Work out the finished part from the listing and answer in its coordinate system (mm). Give positions to 0.01 mm unless a question says otherwise; leave off trailing zeros. Loops run counter-clockwise (first coordinate to the right, second up) from the corner with the lowest first, then second, coordinate; pieces in that order, holes last. Notation, with made-up numbers: (1, 87) - (11, 87) arc R27 cw to (11, 108) - close; hole circle Ø3 at (46.5, -9). An arc over 180 degrees is marked (long way). One line per item, written item: value.
Autodesk Inventor part; units mm, degrees
ref_plane "YZ Plane" through (0, 0, 0) normal (1, 0, 0) x (0, 1, 0)
ref_plane "XZ Plane" through (0, 0, 0) normal (0, 1, 0) x (-1, 0, 0)
ref_plane "XY Plane" through (0, 0, 0) normal (0, 0, 1) x (1, 0, 0)
sketch "Sketch1" plane through (0, 0, 0) normal (0, 0, 1) x (1, 0, 0)
  line L0 (-5.04, 3.6) -> (5.04, 3.6)
  line L1 (5.04, 3.6) -> (5.04, -3.6)
  line L2 (-5.04, -3.6) -> (-5.04, 3.6)
  line L3 (-2.79, -3.4) -> (-2.79, -3.6)
  line L4 (-2.79, -3.6) -> (-2.29, -3.6)
  line L5 (-2.29, -3.6) -> (-2.29, -3.4)
  line L6 (-0.25, -3.4) -> (-0.25, -3.6)
  line L7 (-0.25, -3.6) -> (0.25, -3.6)
  line L8 (0.25, -3.6) -> (0.25, -3.4)
  line L9 (2.29, -3.4) -> (2.29, -3.6)
  line L10 (2.29, -3.6) -> (2.79, -3.6)
  line L11 (2.79, -3.6) -> (2.79, -3.4)
  line L12 (-2.79, -3.4) -> (-4.79, -3.4)
  line L13 (-0.25, -3.4) -> (-2.29, -3.4)
  line L14 (4.79, -3.4) -> (2.79, -3.4)
  line L15 (2.29, -3.4) -> (0.25, -3.4)
  line L16 (0, 1.3653) -> (0, -1.7187) construction
  line L17 (-4.79, -3.4) -> (-4.79, -3.6)
  line L18 (-4.79, -3.6) -> (-5.04, -3.6)
  line L19 (4.79, -3.4) -> (4.79, -3.6)
  line L20 (4.79, -3.6) -> (5.04, -3.6)
  point P0 (0, 0)
  point P1 (0, 3.6)
  point P2 (-5.04, 0)
  point P3 (0, -3.6)
  point P4 (-2.54, -3.6)
  point P5 (-2.54, -3.6)
  point P6 (5.04, 0)
  dimension "d0" = 0.5
  dimension "d1" = 0.2
  dimension "d3" = 10.08
  dimension "d4" = 2.54
  dimension "d20" = 7
  dimension "d21" = 0.25
extrude "Extrusion1" add sketch "Sketch1" along normal blind 2.54
sketch "Sketch3" plane through (-5.04, -3.4, 0) normal (0, -1, 0) x (1, 0, 0)
  line L0 (0.93, 2.87) -> (1.53, 2.87)
  line L1 (1.53, 2.87) -> (1.53, 1.87)
  line L2 (1.53, 1.87) -> (0.93, 1.87)
  line L3 (0.93, 1.87) -> (0.93, 2.87)
  line L4 (0.93, 0.67) -> (1.53, 0.67)
  line L5 (1.53, 0.67) -> (1.53, -0.33)
  line L6 (1.53, -0.33) -> (0.93, -0.33)
  line L7 (0.93, -0.33) -> (0.93, 0.67)
  line L8 (3.47, 2.87) -> (4.07, 2.87)
  line L9 (4.07, 2.87) -> (4.07, 1.87)
  line L10 (4.07, 1.87) -> (3.47, 1.87)
  line L11 (3.47, 1.87) -> (3.47, 2.87)
  line L12 (3.47, 0.67) -> (4.07, 0.67)
  line L13 (4.07, 0.67) -> (4.07, -0.33)
  line L14 (4.07, -0.33) -> (3.47, -0.33)
  line L15 (3.47, -0.33) -> (3.47, 0.67)
  line L16 (6.01, 2.87) -> (6.61, 2.87)
  line L17 (6.61, 2.87) -> (6.61, 1.87)
  line L18 (6.61, 1.87) -> (6.01, 1.87)
  line L19 (6.01, 1.87) -> (6.01, 2.87)
  line L20 (6.01, 0.67) -> (6.61, 0.67)
  line L21 (6.61, 0.67) -> (6.61, -0.33)
  line L22 (6.61, -0.33) -> (6.01, -0.33)
  line L23 (6.01, -0.33) -> (6.01, 0.67)
  line L24 (8.55, 2.87) -> (9.15, 2.87)
  line L25 (9.15, 2.87) -> (9.15, 1.87)
  line L26 (9.15, 1.87) -> (8.55, 1.87)
  line L27 (8.55, 1.87) -> (8.55, 2.87)
  line L28 (8.55, 0.67) -> (9.15, 0.67)
  line L29 (9.15, 0.67) -> (9.15, -0.33)
  line L30 (9.15, -0.33) -> (8.55, -0.33)
  line L31 (8.55, -0.33) -> (8.55, 0.67)
  line L32 (4.79, 0) -> (2.75, 0)
  line L33 (6.0777, 1.27) -> (8.8799, 1.27) construction
  line L34 (0, 0) -> (0, 2.54)
  line L35 (0, 0) -> (0, 2.54)
  point P0 (5.04, 0)
  point P1 (1.23, -0.33)
  point P2 (3.77, -0.33)
  point P3 (6.31, -0.33)
  point P4 (8.85, -0.33)
  point P5 (3.77, -0.33)
  point P6 (1.23, -0.33)
  point P7 (6.31, -0.33)
  point P8 (8.85, -0.33)
  point P9 (3.77, 0)
  point P10 (0, 1.27)
  dimension "d11" = 3.2
  dimension "d12" = 0.6
  dimension "d13" = 2.54
  dimension "d14" = 2.54
  dimension "d15" = 2.54
  dimension "d16" = 1
extrude "Extrusion3" add sketch "Sketch3" along normal blind 0.2
sketch "Sketch5" plane through (-5.04, 3.6, 0) normal (0, 1, 0) x (1, 0, 0)
  line L0 (0, 0) -> (10.08, 0)
  line L1 (0, 0) -> (0, -2.54)
  line L2 (10.08, -2.54) -> (0, -2.54)
  line L3 (10.08, 0) -> (10.08, -2.54)
  line L4 (0.73, -0.77) -> (1.73, -0.77)
  line L5 (1.73, -0.77) -> (1.73, -1.77)
  line L6 (1.73, -1.77) -> (0.73, -1.77)
  line L7 (0.73, -1.77) -> (0.73, -0.77)
  line L8 (1.53, 0.33) -> (0.93, 0.33)
  point P0 (5.04, 0)
  point P1 (0.73, -1.27)
  point P2 (0, -1.27)
  point P3 (1.23, -0.77)
  point P4 (1.23, 0.33)
  dimension "d23" = 1
extrude "Extrusion4" cut sketch "Sketch5" against normal blind 7 contours L4 L5 L6 L7
chamfer "Chamfer1" distance 0.5 angle 45 4 edges at (-3.81, 3.6, 0.77) (-3.31, 3.6, 1.27) (-4.31, 3.6, 1.27) (-3.81, 3.6, 1.77)
pattern_linear "Rectangular Pattern1" count 4 spacing 2.54 along (1, 0, 0) of "Extrusion4", "Chamfer1"
properties part number "fciconnect-91601-304"
1. Section A-A (y = -3) is taken. Write down the section's boundary in (x, z).
Output:
outline: (-5.04, 0) - (5.04, 0) - (5.04, 2.54) - (-5.04, 2.54) - close; hole (-4.31, 0.77) - (-3.31, 0.77) - (-3.31, 1.77) - (-4.31, 1.77) - close; hole (-1.77, 0.77) - (-0.77, 0.77) - (-0.77, 1.77) - (-1.77, 1.77) - close; hole (0.77, 0.77) - (1.77, 0.77) - (1.77, 1.77) - (0.77, 1.77) - close; hole (3.31, 0.77) - (4.31, 0.77) - (4.31, 1.77) - (3.31, 1.77) - close
2. Flat-ended cylindrical pins translate along their axes: pin 1 Ø4 at (x, y) = (3, 2.5) entering from +Z; pin 2 Ø0.6 at (x, z) = (3.5, 1) entering from -Y; pin 3 Ø0.8 at (x, y) = (-1.5, 0) entering from -Z; pin 4 Ø1.6 at (x, z) = (-4, 1.5) entering from -Y. Find the tip coordinate at first contact, or state that the pin passes through.
Output:
pin 1: stops at z = 2.54
pin 2: stops at y = -3.4
pin 3: stops at z = 0
pin 4: stops at y = -3.6
3. The mould has two halves that part along Z. Classify faces 1 (the flat face through (0, 0, 2.54)), 2 (the flat face through (1, 0, 0.77)), 3 (the flat face through (0, 0, 0)): released by +Z, released by -Z, zero draft, split by the parting line, or undercut.
Output:
face 1: released by +Z
face 2: undercut
face 3: released by -Z
4. Section B-B (z = 2.65) is taken. Write down the section's boundary in (x, y), and give its area (3 significant figures).
Output:
outline: (-4.11, -3.6) - (-3.51, -3.6) - (-3.51, -3.4) - (-4.11, -3.4) - close; (-1.57, -3.6) - (-0.97, -3.6) - (-0.97, -3.4) - (-1.57, -3.4) - close; (0.97, -3.6) - (1.57, -3.6) - (1.57, -3.4) - (0.97, -3.4) - close; (3.51, -3.6) - (4.11, -3.6) - (4.11, -3.4) - (3.51, -3.4) - close
area: 0.480 mm²
5. Section C-C (x = -2) is taken. Write down the section's boundary in (y, z), and give its area (3 significant figures).
Output:
outline: (-3.4, 0) - (3.6, 0) - (3.6, 0.27) - (3.33, 0.54) - (3.33, 2) - (3.6, 2.27) - (3.6, 2.54) - (-3.4, 2.54) - close
area: 17.3 mm²
6. Find the intervals of material crossed by line 1 along X through (y, z) = (0.5, 1.25); line 2 along Z through (x, y) = (3.75, 0.5); line 3 along Z through (x, y) = (-0.5, 2), in increasing order.
Output:
line 1: x = -5.04 to -4.31, -3.31 to -1.77, -0.77 to 0.77, 1.77 to 3.31, 4.31 to 5.04
line 2: z = 0 to 0.77, 1.77 to 2.54
line 3: z = 0 to 2.54
7. Section D-D (x = 4) is taken. Write down the section's boundary in (y, z).
Output:
outline: (-3.6, -0.33) - (-3.4, -0.33) - (-3.4, 0) - (3.6, 0) - (3.6, 0.27) - (3.1, 0.77) - (-3.4, 0.77) - (-3.4, 0.67) - (-3.6, 0.67) - close; (-3.6, 1.87) - (-3.4, 1.87) - (-3.4, 1.77) - (3.1, 1.77) - (3.6, 2.27) - (3.6, 2.54) - (-3.4, 2.54) - (-3.4, 2.87) - (-3.6, 2.87) - close
